Here's how the part is built. I have some questions about the finished solid (model axes, mm). Face numbers are marked on the shaded views. A direction names the side the tool comes from. Coordinates: 2 decimals unless noted, no trailing zeros. Loops run counter-clockwise (first coordinate to the right, second up) from the corner with the lowest first, then second, coordinate; pieces in that order, holes last. Notation, with made-up numbers: M -11.75,36.25 L 32.25,36.25 A20 cw 32.25,63.25 Z; hole C -27.75,39 d10. An arc over 180 degrees is marked long. Use CSV: the item, a comma, the result in double quotes. Start each with the question number.
Q1. If we section it at C-C (y = -20): Please give me the cut outline in (x, z), and give its area (3 significant figures).
Q2. Which directions (+Z, -Z, +X, -X, +Y, -Y) give clear straight access to the entire face, cutting with the end or side of a thin tool? Please do the marked faces 1 and 2.
Q3. If we section it at A-A (z = 6): Please give me the cut outline in (x, y).
Q4. For pin 1 Ø10 at (x, y) = (22.5, -10) entering from -Z; pin 2 Ø8 at (x, y) = (15, -25.5) entering from +Z; pin 3 Ø3.5 at (y, z) = (-33.02, 33.47) entering from +X; pin 4 Ø3 at (x, z) = (22.5, 9.5) entering from +Y (3 decimals), each with a flat end and sliding along its axis, tell me the tip position at first contact or that it passes through.
Q5. If we section it at D-D (z = 16.5): Please give me the cut outline in (x, y), and give its area (3 significant figures).
Q6. If we mould it in two halves opening along X, with no side actions, what happens to the marked faces 3, 4 and 5? For each: +X half, -X half, draft (parallel to the pull), parting line (faces both ways), or undercut.
Q7. If we section it at B-B (y = -33.5): Please give me the cut outline in (x, z).
Q8. Please list where these lines run through material, in increasing order: probe 1 along X at (y, z) = (-19.5, 7.5); probe 2 along Z at (x, y) = (20.5, -11); probe 3 along X at (y, z) = (-31, 9). Write a range as [from, to].
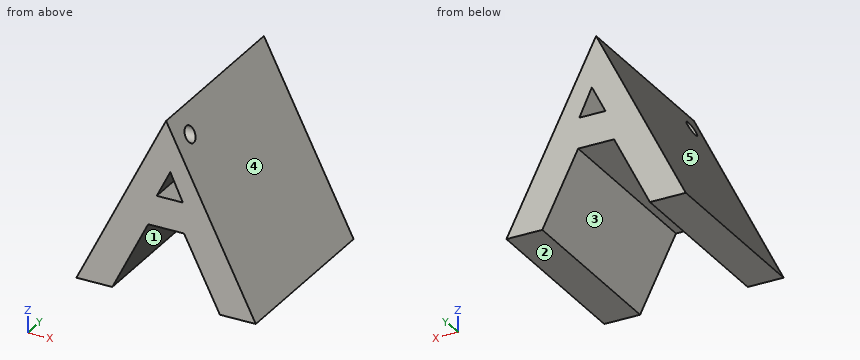
from build123d import *

# Parameters (mm, degrees)
F0_W     = 38.1
F0_H     = 38.1
F1_DEPTH = 38.1
F5_DEPTH = 38.1
F6_R     = 1.5875
F7_DEPTH = 38.1


with BuildPart() as f1:
    # F0 (on Front) → F1 (new body)
    with BuildSketch(Plane.XZ):
        with Locations((19.05, 19.05)):
            Rectangle(F0_W, F0_H)
    extrude(amount=F1_DEPTH)

    # F4 (on offset) → F5 (cut)
    with BuildSketch(Plane.XZ.offset(38.1)):
        Polygon((19.05, 38.1), (0, 38.1), (0, 0), align=None)
        Polygon((22.606704, 21.720167), (19.947089, 27.482659), (17.065844, 21.720167), align=None)
        Polygon((15.24, 15.24), (7.62, 0), (30.48, 0), (22.86, 15.24), align=None)
        Polygon((38.1, 38.1), (19.05, 38.1), (38.1, 0), align=None)
    extrude(amount=-F5_DEPTH, mode=Mode.SUBTRACT)

    # F6 (on offset) → F7 (cut)
    with BuildSketch(Plane.YZ.offset(38.1)):
        with Locations((-33.023518, 33.466786)):
            Circle(F6_R)
    extrude(amount=-F7_DEPTH, mode=Mode.SUBTRACT)


solid = f1.part
Results below:
1,outline,"M 0,0 L 7.62,0 L 15.24,15.24 L 22.86,15.24 L 30.48,0 L 38.1,0 L 19.05,38.1 Z; hole M 17.07,21.72 L 22.61,21.72 L 19.95,27.48 Z"
1,area,"478 mm^2"
2,face 1,"-Z, +Y, -Y"
2,face 2,"-Z, +X, -X, +Y, -Y"
3,outline,"M 3,-38.1 L 10.62,-38.1 L 10.62,0 L 3,0 Z; M 27.48,-38.1 L 35.1,-38.1 L 35.1,0 L 27.48,0 Z"
4,pin 1,"z = 5.96"
4,pin 2,"z = 38"
4,pin 3,"x = 22.24"
4,pin 4,"through"
5,outline,"M 8.25,-38.1 L 29.85,-38.1 L 29.85,0 L 8.25,0 Z"
5,area,"823 mm^2"
6,face 3,"undercut"
6,face 4,"+X half"
6,face 5,"-X half"
7,outline,"M 0,0 L 7.62,0 L 15.24,15.24 L 22.86,15.24 L 30.48,0 L 38.1,0 L 22.12,31.95 L 15.98,31.95 Z; M 17.49,34.98 L 20.61,34.98 L 19.05,38.1 Z; hole M 17.07,21.72 L 22.61,21.72 L 19.95,27.48 Z"
8,probe 1,"[3.75, 11.37], [26.73, 34.35]"
8,probe 2,"[15.24, 21.72], [26.28, 35.2]"
8,probe 3,"[4.5, 12.12], [25.98, 33.6]"
